from build123d import *

# Parameters (mm, degrees)
EXTRUDE1_DEPTH = 22.86
CHAMFER1_SIZE  = 0.254
CHAMFER3_SIZE  = 0.762
CHAMFER4_SIZE  = 0.762
FILLET1_R      = 0.508


with BuildPart() as part:
    # Sketch1 → Extrude1 (new body)
    with BuildSketch(Plane(origin=(0, 0, 0), x_dir=(0, 0, -1), z_dir=(1, 0, 0))):
        Polygon((9.165435523, 15.875), (-9.165435523, 15.875), (-18.330871047, 0), (-9.165435523, -15.875), (9.165435523, -15.875), (18.330871047, 0), align=None)
    extrude(amount=EXTRUDE1_DEPTH)

    # Sketch2 → Cut-Revolve1 (revolve, cut)
    with BuildSketch(Plane.XY, mode=Mode.PRIVATE) as cut_revolve1_sk:
        Polygon((0, 12.2555), (0, 0), (22.86, 0), (22.86, 8.255), (22.606, 8.255), (22.606, 4.953), (22.479, 4.926005317), (21.858294683, 4.3053), (15.24, 4.3053), (14.478, 5.0673), (14.478, 11.7221), (10.16, 11.7221), (10.16, 12.2555), align=None)
    revolve(cut_revolve1_sk.sketch.rotate(Axis((0, 0, 0), (1, 0, 0)), 270), axis=Axis((0, 0, 0), (1, 0, 0)), mode=Mode.SUBTRACT)  # turned: the seam where the file's is

    # Chamfer1
    chamfer1_edges = [part.edges().sort_by_distance(p)[0] for p in [
        (0, 0, 12.2555),
    ]]
    chamfer(chamfer1_edges, length=CHAMFER1_SIZE)

    # Chamfer3
    chamfer3_edges = [part.edges().sort_by_distance(p)[0] for p in [
        (0, -7.9375, -13.748153285),
        (0, -15.875, 0),
        (0, -7.9375, 13.748153285),
        (0, 7.9375, 13.748153285),
        (0, 15.875, 0),
        (0, 7.9375, -13.748153285),
    ]]
    chamfer(chamfer3_edges, length=CHAMFER3_SIZE)

    # Chamfer4
    chamfer4_edges = [part.edges().sort_by_distance(p)[0] for p in [
        (22.86, 7.9375, 13.748153285),
        (22.86, -7.9375, 13.748153285),
        (22.86, -15.875, 0),
        (22.86, -7.9375, -13.748153285),
        (22.86, 7.9375, -13.748153285),
        (22.86, 15.875, 0),
    ]]
    chamfer(chamfer4_edges, length=CHAMFER4_SIZE)

    # Fillet1
    fillet1_edges = [part.edges().sort_by_distance(p)[0] for p in [
        (10.16, 0, 12.2555),
    ]]
    fillet(fillet1_edges, radius=FILLET1_R)


solid = part.part
Here's how the part is built. I have some questions about the finished solid (model axes, mm). A direction names the side the tool comes from. Round coordinates to 2 decimals unless told otherwise and drop trailing zeros. Loops run counter-clockwise (first coordinate to the right, second up) from the corner with the lowest first, then second, coordinate; pieces in that order, holes last. Notation, with made-up numbers: (-17, -19) -> (10, -19) arc R20 ccw to (10, 19) -> close; hole circle Ø10 at (2.25, -30.5). An arc over 180 degrees is marked (long way). Write each question's results on one line, items separated by ' | '.
(1) For faces 1 (the face through (14.478, -5, 2)), 2 (the face through (0.39, 7.64, -13.49)), 3 (the face through (22.606, -4, -4)), which set-ups out of +Z, -Z, +X, -X, +Y, -Y let a thin tool reach every point of the face, with its end or its side?
Worked answers:
face 1: -X | face 2: -Z, -X, +Y | face 3: +X
(2) For P1, Ø2, axis at x = 3, z = -14.5, coming from the -Y side; P2, Ø8, axis at x = 5.5, y = 10, coming from the -Z side; P3, Ø1, axis at x = 17.5, y = -1, coming from the +Z side, each with a flat end and sliding along its axis, tell me the tip position at first contact or that it passes through.
Worked answers:
P1: y = -8.37 | P2: z = -14.87 | P3: z = 18.04
(3) If I drill on L1, parallel to Y at x = 18.25, z = 0 (3 decimals); L2, parallel to X at y = -5.5, z = 0.5; L3, parallel to Y at x = 11.4, z = 0 (3 decimals), over which ranges is the centre line in solid material (lowest first)?
Worked answers:
L1: -15.875 to -4.305, 4.305 to 15.875 | L2: 14.48 to 22.61 | L3: -15.875 to -11.722, 11.722 to 15.875
(4) If we section it at B-B, the plane x = 2: List the corners of the cut face in (y, z) for me (1 decimal).
Worked answers:
outline: (-15.9, -9.2) -> (0, -18.3) -> (15.9, -9.2) -> (15.9, 9.2) -> (0, 18.3) -> (-15.9, 9.2) -> close; hole circle Ø24.5 at (0, 0)
(5) If we section it at C-C, the plane z = 16.5: List the corners of the cut face in (x, y) for me.
Worked answers:
outline: (0, -1.65) -> (0.76, -3.17) -> (22.1, -3.17) -> (22.86, -1.65) -> (22.86, 1.65) -> (22.1, 3.17) -> (0.76, 3.17) -> (0, 1.65) -> close
(6) If we section it at D-D, the plane x = 10.75: List the corners of the cut face in (y, z) for me (3 decimals).
Worked answers:
outline: (-15.875, -9.165) -> (0, -18.331) -> (15.875, -9.165) -> (15.875, 9.165) -> (0, 18.331) -> (-15.875, 9.165) -> close; hole circle Ø23.444 at (0, 0)
(7) We'd pull the mould along Y, two halves only. Please class faces 4 (the face through (12.289, -11.443, 2.541)), 5 (the face through (11.28, 7.83, -13.81)), 6 (the face through (0.39, -7.64, 13.49)): released by +Y, released by -Y, zero draft, split by the parting line, or undercut.
Worked answers:
face 4: undercut | face 5: released by +Y | face 6: released by -Y
